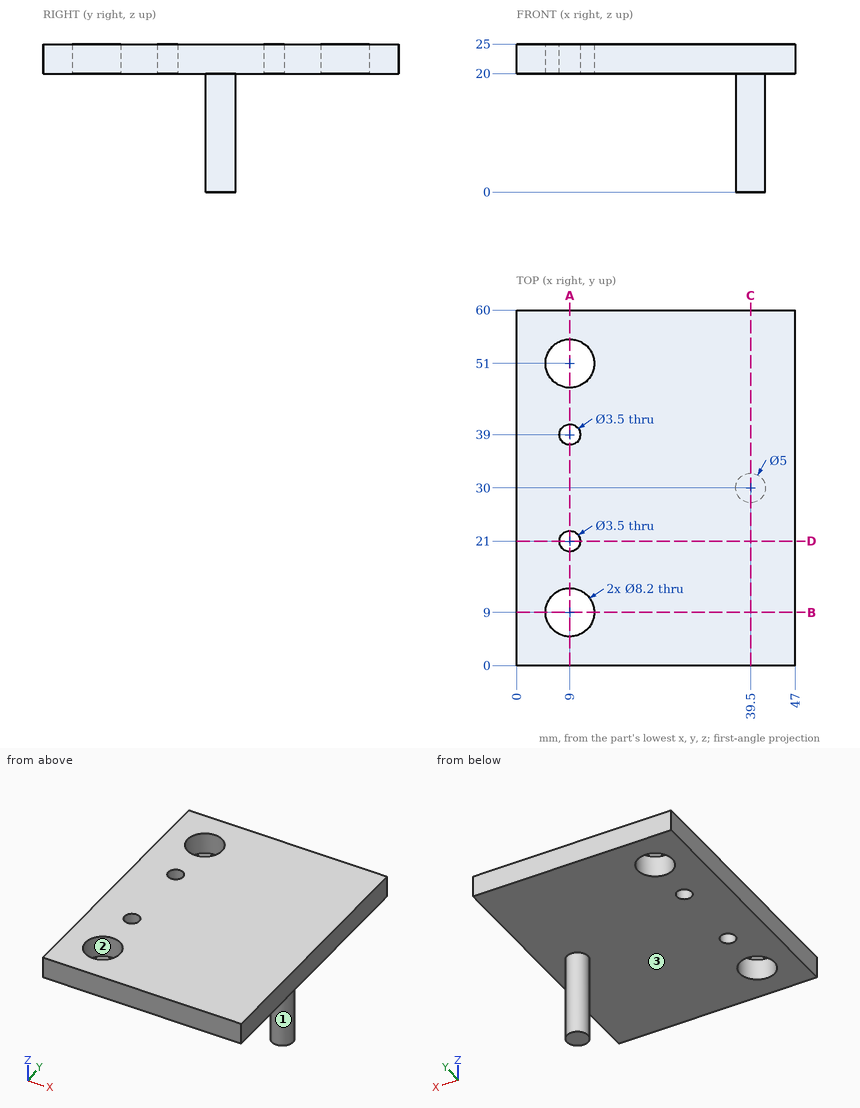
Drawing for the job (mm, zero at the part's lowest x, y, z). Coordinates: 2 decimals unless noted, no trailing zeros. Order: outer loops, then holes, each group sorted by start corner. A loop starts at its lowest first (then second) coordinate and runs counter-clockwise, first axis right, second up. Notation, with made-up numbers: (-4, 12.5) - (1, 12.5) arc R26 ccw to (1, 37.5) - close; hole circle Ø9 at (26, 20). An arc over 180 degrees is marked (long way). Use a Markdown table: item, result. Add a question column.
(1) Saw through at A-A (x = 9). Give the cut face in (y, z).
(2) Drill centre lines: line 1 along Y through (x, z) = (9, 22.3); line 2 along Z through (x, y) = (41.5, 43); line 3 along Y through (x, z) = (37.5, 19). Where is each one in solid material? Low to high. Write a range as [from, to].
(3) Saw through at B-B (y = 9). Give the cut face in (x, z).
(4) Saw through at C-C (x = 39.5). Give the cut face in (y, z), then the cut area to 3 significant figures.
(5) Saw through at D-D (y = 21). Give the cut face in (x, z), then the cut area to 4 significant figures.
(6) Pull direction X, two halves, no side cores. Call the marked faces 1, 2 and 3: +X half, -X half, draft (parallel to the pull), parting line (faces both ways), or undercut.
(7) Flat gauge pins, fed straight in: pin 1 (8 mm diameter, centred on y = 24, z = 14, fed in from +X); pin 2 (10 mm diameter, centred on x = 13, y = 53, fed in from -Z); pin 3 (7.5 mm diameter, centred on x = 9, y = 9, fed in from +Z); pin 4 (5 mm diameter, centred on x = 6, z = 18.5, fed in from +Y). Where does each tip first touch, or does it go through?
Solved:
| question | item | result |
|---|---|---|
| 1 | outline | (0, 20) - (4.9, 20) - (4.9, 25) - (0, 25) - close; (13.1, 20) - (19.25, 20) - (19.25, 25) - (13.1, 25) - close; (22.75, 20) - (37.25, 20) - (37.25, 25) - (22.75, 25) - close; (40.75, 20) - (46.9, 20) - (46.9, 25) - (40.75, 25) - close; (55.1, 20) - (60, 20) - (60, 25) - (55.1, 25) - close |
| 2 | line 1 | y = [0, 4.9], [13.1, 19.25], [22.75, 37.25], [40.75, 46.9], [55.1, 60] |
| 2 | line 2 | z = [20, 25] |
| 2 | line 3 | y = [28.5, 31.5] |
| 3 | outline | (0, 20) - (4.9, 20) - (4.9, 25) - (0, 25) - close; (13.1, 20) - (47, 20) - (47, 25) - (13.1, 25) - close |
| 4 | outline | (0, 20) - (27.5, 20) - (27.5, 0) - (32.5, 0) - (32.5, 20) - (60, 20) - (60, 25) - (0, 25) - close |
| 4 | area | 400 mm² |
| 5 | outline | (0, 20) - (7.25, 20) - (7.25, 25) - (0, 25) - close; (10.75, 20) - (47, 20) - (47, 25) - (10.75, 25) - close |
| 5 | area | 217.5 mm² |
| 6 | face 1 | parting line |
| 6 | face 2 | undercut |
| 6 | face 3 | draft |
| 7 | pin 1 | stops at x = 41 |
| 7 | pin 2 | stops at z = 20 |
| 7 | pin 3 | passes through |
| 7 | pin 4 | stops at y = 60 |
